Verification items for the finished model (mm, model axes). A direction names the side the tool comes from. Round coordinates to 2 decimals unless told otherwise and drop trailing zeros. Write each loop counter-clockwise with the first axis right and the second up, starting at its lowest first coordinate (ties: lowest second). Pieces come first, ordered by that corner, then holes. Notation, with made-up numbers: (-18.5, -22.5) - (6.5, -22.5) arc R15 ccw to (6.5, -2.5) - close; hole circle Ø3 at (13, -22). An arc over 180 degrees is marked (long way). Write each question's results on one line, items separated by ' | '.
```python
from build123d import *

# Parameters (mm, degrees)
SKETCH_1_W          = 100
SKETCH_1_H          = 30
EXTRUDE_1_DEPTH     = 5
SKETCH_2_R          = 1.6
CUT_EXTRUDE_1_DEPTH = 5
SKETCH_3_W          = 20
SKETCH_3_H          = 20
EXTRUDE_2_DEPTH     = 16
SKETCH_4_W          = 13
SKETCH_4_H          = 13
CUT_EXTRUDE_2_DEPTH = 16
SKETCH_5_R          = 2.5
CUT_EXTRUDE_3_DEPTH = 10


with BuildPart() as part:
    # Эскиз1 → Бобышка-Вытянуть1 (new body)
    with BuildSketch(Plane(origin=(0, 0, 0), x_dir=(1, 0, 0), z_dir=(0, 1, 0))):
        with Locations((10.328317373, 5.793433653)):
            Rectangle(SKETCH_1_W, SKETCH_1_H)
    extrude(amount=EXTRUDE_1_DEPTH)

    # Эскиз2 → Вырез-Вытянуть1 (cut)
    with BuildSketch(Plane(origin=(0, 5, 0), x_dir=(1, 0, 0), z_dir=(0, 1, 0))):
        with Locations(Location((-34.671682627, 15.893433653, 0), (0, 0, 270))):
            Circle(SKETCH_2_R)
        with Locations(Location((-34.671682627, -4.306566347, 0), (0, 0, 270))):
            Circle(SKETCH_2_R)
        with Locations(Location((55.328317373, 15.893433653, 0), (0, 0, 270))):
            Circle(SKETCH_2_R)
        with Locations(Location((55.328317373, -4.306566347, 0), (0, 0, 270))):
            Circle(SKETCH_2_R)
    extrude(amount=-CUT_EXTRUDE_1_DEPTH, mode=Mode.SUBTRACT)

    # Эскиз3 → Бобышка-Вытянуть2 (add)
    with BuildSketch(Plane.XZ):
        with Locations((10.328317373, -5.793433653)):
            Rectangle(SKETCH_3_W, SKETCH_3_H)
    extrude(amount=EXTRUDE_2_DEPTH)

    # Эскиз4 → Вырез-Вытянуть2 (cut)
    with BuildSketch(Plane.XZ.offset(16)):
        with Locations((10.328317373, -5.793433653)):
            Rectangle(SKETCH_4_W, SKETCH_4_H)
    extrude(amount=-CUT_EXTRUDE_2_DEPTH, mode=Mode.SUBTRACT)

    # Эскиз5 → Вырез-Вытянуть3 (cut)
    with BuildSketch(Plane(origin=(20.328317373, 0, 0), x_dir=(0, 0, -1), z_dir=(1, 0, 0))):
        with Locations((5.793433653, -7)):
            Circle(SKETCH_5_R)
    extrude(amount=-CUT_EXTRUDE_3_DEPTH, mode=Mode.SUBTRACT)


solid = part.part
```
(1) Mould release check, pull along Z, two halves, no side actions. Record for faces 1 (the flat face through (10, -8, 4.207)), 2 (the flat face through (10, 0, -16)), 3 (the cylindrical face through (56.915, 2.535, 4.098)): released by +Z, released by -Z, zero draft, split by the parting line, or undercut.
Answer:
face 1: released by +Z | face 2: zero draft | face 3: undercut
(2) Set-up check for faces 4 (the flat face through (10, -8, -15.793)), 5 (the flat face through (20.328, -10, -6)), 6 (the flat face through (3.828, -8, -6)): record each of +Z, -Z, +X, -X, +Y, -Y from which the full face is reachable in a straight line by a thin tool's end or side.
Answer:
face 4: -Z, +X, -X, -Y | face 5: +Z, -Z, +X, -Y | face 6: -Y
(3) Section check A-A (y = -3.5). Record the cut outline in (x, z), plus the area to 3 significant figures.
Answer:
outline: (0.33, -15.79) - (20.33, -15.79) - (20.33, 4.21) - (0.33, 4.21) - close; hole (3.83, -12.29) - (16.83, -12.29) - (16.83, 0.71) - (3.83, 0.71) - close | area: 231 mm2
(4) Thickness scan on L1, parallel to X at y = -10, z = -2.25; L2, parallel to Z at x = 14.5, y = -2.25; L3, parallel to Y at x = 44.5, z = -10. Record the ranges inside material, lowest first.
Answer:
L1: 0.33 to 3.83, 16.83 to 20.33 | L2: -15.79 to -12.29, 0.71 to 4.21 | L3: 0 to 5
(5) Section check C-C (x = 49). Record the cut outline in (y, z).
Answer:
outline: (0, -20.79) - (5, -20.79) - (5, 9.21) - (0, 9.21) - close
(6) Section check B-B (x = 15). Record the cut outline in (y, z), plus the area to 3 significant figures.
Answer:
outline: (-16, -15.79) - (0, -15.79) - (0, -20.79) - (5, -20.79) - (5, 9.21) - (0, 9.21) - (0, 4.21) - (-16, 4.21) - (-16, 0.71) - (0, 0.71) - (0, -12.29) - (-16, -12.29) - close | area: 262 mm2
(7) Go/stop test with flat-tipped pins: pin 1 Ø6.5 at (y, z) = (-11.5, -7.5) entering from -X; pin 2 Ø6.5 at (x, z) = (9, -6.5) entering from -Y; pin 3 Ø8 at (x, y) = (9.5, -5) entering from -Z; pin 4 Ø1.9 at (x, z) = (-34.67, -15.89) entering from -Y. Record where each tip stops, or that it passes through.
Answer:
pin 1: x = 0.33 | pin 2: y = 0 | pin 3: z = -15.79 | pin 4: through
